Answer from the drawing. Dimensions are ordinates in mm from the lowest x, y and z of the part. Coordinates: 2 decimals unless noted, no trailing zeros. Write each loop counter-clockwise with the first axis right and the second up, starting at its lowest first coordinate (ties: lowest second). Pieces come first, ordered by that corner, then holes. Notation, with made-up numbers: (6, 71) -> (56, 71) arc R3 cw to (56, 76) -> close; hole circle Ø6 at (24.5, -20). An arc over 180 degrees is marked (long way). Answer as a JSON object with one key per item and string values. Group by question number.
(1) Find section C-C (y = 3.65). Give the vertices of the cut face in (x, z).
(2) Find section A-A (z = 17.5). Give the vertices of the cut face in (x, y).
(3) Straight lines are drawn through the part: L1, parallel to X at y = 0.45, z = 18; L2, parallel to X at y = 0.75, z = 50; L3, parallel to X at y = 4.3, z = 49.5. For each, find the intervals that lie inside material, in ascending order.
(4) A flat-ended cylindrical pin translates along its axis: P1, Ø3.5, axis at x = 52.5, z = 47.81, coming from the -Y side. Find the tip coordinate at first contact, or state that the pin passes through.
(5) Find section B-B (x = 35). Give the vertices of the cut face in (y, z), then the cut area to 3 significant figures.
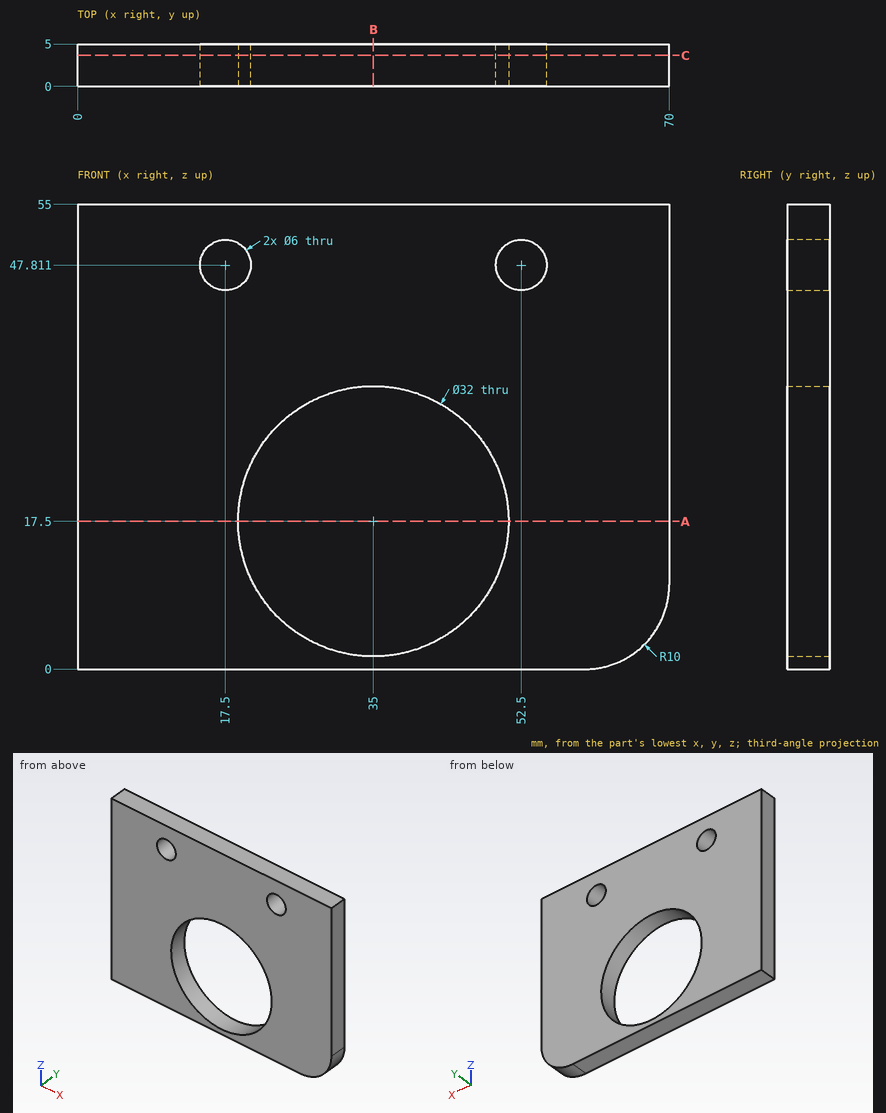
Results below:
{
 "1": {"outline": "(0, 0) -> (60, 0) arc R10 ccw to (70, 10) -> (70, 55) -> (0, 55) -> close; hole circle Ø6 at (17.5, 47.81); hole circle Ø32 at (35, 17.5); hole circle Ø6 at (52.5, 47.81)"},
 "2": {"outline": "(0, 0) -> (19, 0) -> (19, 5) -> (0, 5) -> close; (51, 0) -> (70, 0) -> (70, 5) -> (51, 5) -> close"},
 "3": {"L1": "x = 0 to 19.01, 50.99 to 70", "L2": "x = 0 to 15.45, 19.55 to 50.45, 54.55 to 70", "L3": "x = 0 to 15.02, 19.98 to 50.02, 54.98 to 70"},
 "4": {"P1": "passes through"},
 "5": {"outline": "(0, 0) -> (5, 0) -> (5, 1.5) -> (0, 1.5) -> close; (0, 33.5) -> (5, 33.5) -> (5, 55) -> (0, 55) -> close", "area": "115 mm2"}
}
